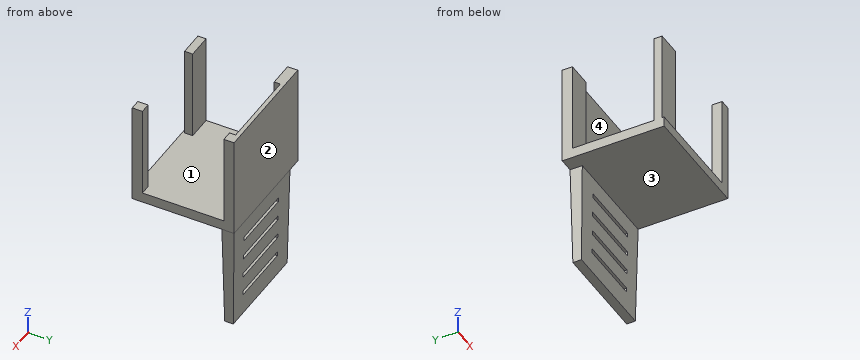
from build123d import *

# Parameters (mm, degrees)
SKETCH1_W           = 500
SKETCH1_H           = 500
BOSS_EXTRUDE1_DEPTH = 50
SKETCH2_W           = 50
SKETCH2_H           = 50
BOSS_EXTRUDE2_DEPTH = 450
SKETCH3_W           = 400
SKETCH3_H           = 20
BOSS_EXTRUDE3_DEPTH = 450
SKETCH4_W           = 500
SKETCH4_H           = 60
BOSS_EXTRUDE4_DEPTH = 509
BOSS_EXTRUDE4_TAPER = 1
SKETCH5_W           = 310
SKETCH5_H           = 21.323695684
CUT_EXTRUDE1_DEPTH  = 509
BOSS_EXTRUDE5_DEPTH = 70
SKETCH7_W           = 120
SKETCH7_H           = 450
CUT_EXTRUDE2_DEPTH  = 10


with BuildPart() as part:
    # Sketch1 → Boss-Extrude1 (new body)
    with BuildSketch(Plane.XY):
        with Locations((-6.756756757, -117.398648649)):
            Rectangle(SKETCH1_W, SKETCH1_H)
    extrude(amount=BOSS_EXTRUDE1_DEPTH)

    # Sketch2 → Boss-Extrude2 (add)
    with BuildSketch(Plane.XY.offset(50)):
        with Locations((-231.756756757, 107.601351351)):
            Rectangle(SKETCH2_W, SKETCH2_H)
        with Locations((218.243243243, 107.601351351)):
            Rectangle(SKETCH2_W, SKETCH2_H)
        with Locations((218.243243243, -342.398648649)):
            Rectangle(SKETCH2_W, SKETCH2_H)
        with Locations((-231.756756757, -342.398648649)):
            Rectangle(SKETCH2_W, SKETCH2_H)
    extrude(amount=BOSS_EXTRUDE2_DEPTH)

    # Sketch3 → Boss-Extrude3 (add)
    with BuildSketch(Plane.XY.offset(50)):
        with Locations((-6.756756757, 122.601351351)):
            Rectangle(SKETCH3_W, SKETCH3_H)
    extrude(amount=BOSS_EXTRUDE3_DEPTH)

    # Sketch4 → Boss-Extrude4 (add)
    with BuildSketch(Plane(origin=(0, 0, 0), x_dir=(-1, 0, 0), z_dir=(0, 0, -1))):
        with Locations((6.756756757, 102.601351351)):
            Rectangle(SKETCH4_W, SKETCH4_H)
    extrude(amount=BOSS_EXTRUDE4_DEPTH, taper=BOSS_EXTRUDE4_TAPER)

    # Sketch5 → Cut-Extrude1 (cut)
    with BuildSketch(Plane(origin=(0, 72.579237961, 1.266875311), x_dir=(1, 0, 0), z_dir=(0, -0.9998476951563913, -0.01745240643728355))):
        with Locations((-2.218768488, -397.78694869)):
            Rectangle(SKETCH5_W, SKETCH5_H)
        with Locations((-2.218768488, -297.78694869)):
            Rectangle(SKETCH5_W, SKETCH5_H)
        with Locations((-2.218768488, -197.78694869)):
            Rectangle(SKETCH5_W, SKETCH5_H)
        with Locations((-2.218768488, -97.78694869)):
            Rectangle(SKETCH5_W, SKETCH5_H)
    extrude(amount=-CUT_EXTRUDE1_DEPTH, mode=Mode.SUBTRACT)

    # Sketch6 → Boss-Extrude5 (add)
    with BuildSketch(Plane.ZY.offset(256.756756757)):
        Polygon((500, 132.601351351), (0, 132.601351351), (0, -367.398648649), (500, -367.398648649), (500, -317.398648649), (50, -317.398648649), (50, 82.601351351), (500, 82.601351351), align=None)
    extrude(amount=BOSS_EXTRUDE5_DEPTH)

    # Sketch7 → Cut-Extrude2 (cut)
    with BuildSketch(Plane.XZ.offset(367.398648649)):
        with Locations((-266.756756757, 275)):
            Rectangle(SKETCH7_W, SKETCH7_H)
    extrude(amount=-CUT_EXTRUDE2_DEPTH, mode=Mode.SUBTRACT)


solid = part.part
Input: part model. Units: mm. Frame: model coordinates. Face numbers are marked on the shaded views. Coordinates: 2 decimals unless noted, no trailing zeros. Write each loop counter-clockwise with the first axis right and the second up, starting at its lowest first coordinate (ties: lowest second). Pieces come first, ordered by that corner, then holes. Notation, with made-up numbers: M 52.5,49 L 81.5,49 A24 ccw 81.5,69 Z; hole C -24.75,-4 d5. An arc over 180 degrees is marked long. Answer as a JSON object with one key per item and string values. Group by question number.
(1) Section A-A on z = 104. Output: boundary loops of the cut face in (x, y).
(2) Section B-B on x = -6. Give the number of separate pieces and of enclosed holes in the cut face, plus the area to 3 significant figures.
(3) Section C-C on y = 43. Output: boundary loops of the cut face in (x, z).
(4) Ray query, line 1 along Y through (x, z) = (-297.5, 439.5); line 2 along Z through (x, y) = (-77.5, 30.5); line 3 along Y through (x, z) = (134, 157.5). Return the intervals inside material, ascending. Write a range as [from, to].
(5) Mould query, pull axis Y, two halves, no side actions, for the marked faces 1, 2, 3 and 4. Classes: pulls with the +Y half, pulls with the -Y half, needs draft (parallel to the pull), parting line crosses it, or undercut.
(6) Contact query for flat-ended pins moving along their axis: P1, Ø5, axis at x = -233, z = 356.5, coming from the -Y side; P2, Ø6.5, axis at y = 96.5, z = -192, coming from the -X side; P3, Ø6.5, axis at y = 101, z = -291, coming from the -X side. Output: stop coordinate, or through.
Result set:
{
 "1": {"outline": "M -326.76,-357.4 L -206.76,-357.4 L -206.76,-317.4 L -326.76,-317.4 Z; M -326.76,82.6 L -206.76,82.6 L -206.76,112.6 L 193.24,112.6 L 193.24,82.6 L 243.24,82.6 L 243.24,132.6 L -326.76,132.6 Z; M 193.24,-367.4 L 243.24,-367.4 L 243.24,-317.4 L 193.24,-317.4 Z"},
 "2": {"separate pieces": "5", "enclosed holes": "0", "area": "55,600 mm2"},
 "3": {"outline": "M -326.76,0 L 243.24,0 L 243.24,50 L -326.76,50 Z"},
 "4": {"line 1": "y = [-357.4, -317.4], [82.6, 132.6]", "line 2": "z = [0, 50]", "line 3": "y = [112.6, 132.6]"},
 "5": {"face 1": "undercut", "face 2": "pulls with the +Y half", "face 3": "needs draft", "face 4": "pulls with the -Y half"},
 "6": {"P1": "stops at y = -357.4", "P2": "stops at x = -253.46", "P3": "stops at x = -251.73"}
}
